Read the model definition and answer for the solid it produces. Units are mm, in the model's axes. A direction names the side the tool comes from. Give positions to 0.01 mm unless a question says otherwise; leave off trailing zeros. Write each loop counter-clockwise with the first axis right and the second up, starting at its lowest first coordinate (ties: lowest second). Pieces come first, ordered by that corner, then holes. Notation, with made-up numbers: (-12, -19) -> (27, -19) arc R15 ccw to (27, -15) -> close; hole circle Ø4 at (-3.75, 56). An arc over 180 degrees is marked (long way). Answer as CSV lines item,"result". Start each with the question number.
1. A tool of negligible diameter and unlimited length cuts with its end or side. For faces 1 (the cylindrical face through (2.944, -1.252, 7.101)), 2 (the flat face through (3, -2.54, 3)), from which of +Z, -Z, +X, -X, +Y, -Y can it reach the whole face along a straight path? Write none if from no direction.
2. Find the intervals of material crossed by line 1 (Z direction, x = 0, y = -5.4); line 2 (Z direction, x = 6.25, y = 1); line 3 (X direction, y = -1, z = 4.5), in increasing order.
3. For a pull along Z with two mould halves and no side action, classify faces 3 (the flat face through (0, -7.938, -3)), 4 (the conical face through (3.805, 11.348, -0.845)), 5 (the cylindrical face through (-2.435, -5.523, 0.767)), 6 (the conical face through (0.423, -1.908, 0.133)) as pulls with the +Z half, pulls with the -Z half, needs draft (parallel to the pull), parting line crosses it, or undercut.
4. The part is cut by section A-A, the plane y = -6. Determine the outline of the cut face in (x, z), and give its area (3 significant figures).
5. Given pin 1 (1.5 mm diameter, centred on y = 2, z = 2.5, fed in from +X); pin 2 (1 mm diameter, centred on x = -3, y = 11, fed in from -Z); pin 3 (3 mm diameter, centred on x = 5, y = 6, fed in from +Z), each flat-ended and moving along its own axis, determine where each tip first touches the part or whether it passes through.
6. The part is cut by section B-B, the plane y = 16. Determine the outline of the cut face in (x, z), and give its area (3 significant figures).
from build123d import *

# Parameters (mm, degrees)
F0_R     = 3.96875
F1_DEPTH = 7.9375
F3_D     = 5.1054
F3_DEPTH = 4.7625
F3_TIP   = 1.5338169022
F6_DEPTH = 2.54


with BuildPart() as f1:
    # F0 (on Front) → F1 (new body)
    with BuildSketch(Plane.XZ):
        Circle(F0_R)
    extrude(amount=F1_DEPTH)

    # F3
    with Locations(Plane.XZ.offset(7.9375)):
        with Locations((0, 0)):
            Hole(F3_D / 2, depth=F3_DEPTH)
            with Locations((0, 0, -(F3_DEPTH + F3_TIP / 2))):  # 118° drill point
                Cone(0, F3_D / 2, F3_TIP, mode=Mode.SUBTRACT)

    # F4 (on Right) → F5 (revolve)
    with BuildSketch(Plane.YZ):
        Polygon((0, 7.68720332), (0, 0), (23.01875, 0), align=None)
    revolve(axis=Axis((0, 11.509375, 0), (0, -1, 0)))

    # F6 (add): a face of the model
    f6_faces = [f1.faces().sort_by_distance(p)[0] for p in [
        (0, 0, -7.4697763762),
    ]]
    extrude(f6_faces, amount=F6_DEPTH)


solid = f1.part
Results found:
1,face 1,"+Y, -Y"
1,face 2,"-Y"
2,line 1,"z = -3.97 to -2.55, 2.55 to 3.97"
2,line 2,"z = -3.87 to 3.87"
2,line 3,"x = -6.23 to 6.23"
3,face 3,"needs draft"
3,face 4,"parting line crosses it"
3,face 5,"undercut"
3,face 6,"undercut"
4,outline,"circle Ø7.94 at (0, 0); hole circle Ø5.11 at (0, 0)"
4,area,"29.0 mm²"
5,pin 1,"stops at x = 6.92"
5,pin 2,"stops at z = -3.19"
5,pin 3,"stops at z = 4.64"
6,outline,"circle Ø4.69 at (0, 0)"
6,area,"17.3 mm²"
